Answer from the drawing. Dimensions are ordinates in mm from the lowest x, y and z of the part. Give positions to 0.01 mm unless a question says otherwise; leave off trailing zeros. Order: outer loops, then holes, each group sorted by start corner. A loop starts at its lowest first (then second) coordinate and runs counter-clockwise, first axis right, second up.
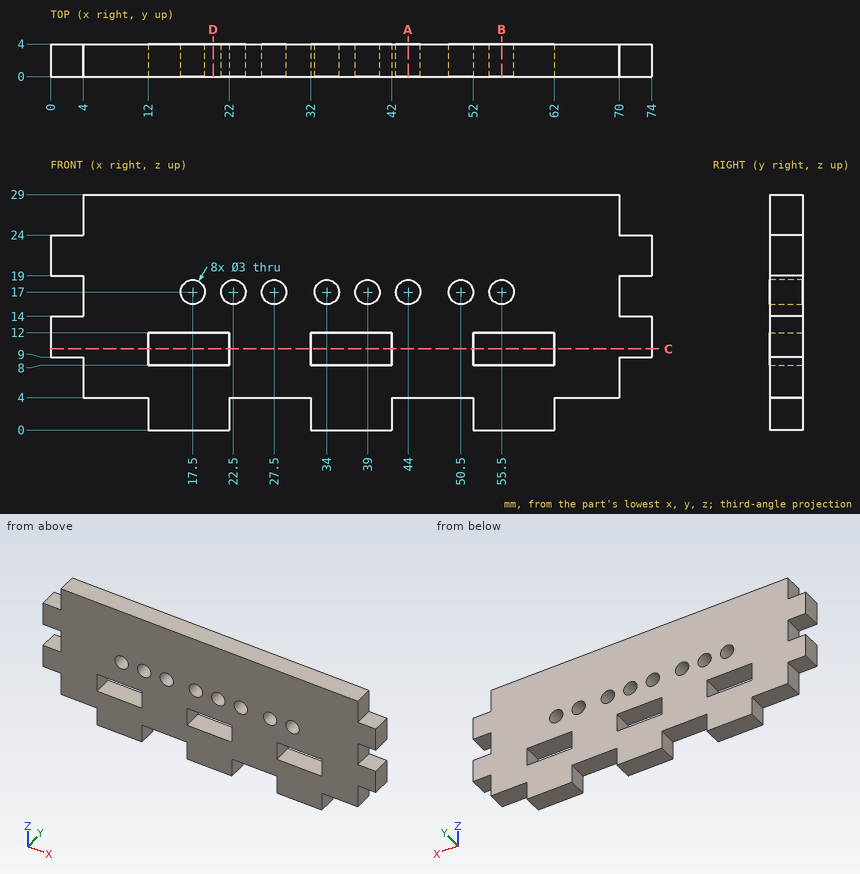
1. Straight lines are drawn through the part: probe 1 along X at (y, z) = (2, 10.75); probe 2 along Z at (x, y) = (61.5, 0.75); probe 3 along Z at (x, y) = (40, 2.75). For each, find the intervals that lie inside material, in ascending order.
Findings below:
probe 1: x = 0 to 12, 22 to 32, 42 to 52, 62 to 74
probe 2: z = 0 to 8, 12 to 29
probe 3: z = 0 to 8, 12 to 15.88, 18.12 to 29
2. The part is cut by section B-B (x = 55.5). Write down the section's boundary in (y, z), then the cut area to 3 significant figures.
Findings below:
outline: (0, 0) - (4, 0) - (4, 8) - (0, 8) - close; (0, 12) - (4, 12) - (4, 15.5) - (0, 15.5) - close; (0, 18.5) - (4, 18.5) - (4, 29) - (0, 29) - close
area: 88.0 mm2
3. The part is cut by section A-A (x = 44). Write down the section's boundary in (y, z).
Findings below:
outline: (0, 4) - (4, 4) - (4, 15.5) - (0, 15.5) - close; (0, 18.5) - (4, 18.5) - (4, 29) - (0, 29) - close
4. The part is cut by section C-C (z = 10). Write down the section's boundary in (x, y), then the cut area to 3 significant figures.
Findings below:
outline: (0, 0) - (12, 0) - (12, 4) - (0, 4) - close; (22, 0) - (32, 0) - (32, 4) - (22, 4) - close; (42, 0) - (52, 0) - (52, 4) - (42, 4) - close; (62, 0) - (74, 0) - (74, 4) - (62, 4) - close
area: 176 mm2
5. Given P1, Ø2.5, axis at x = 17.5, z = 17, coming from the -Y side; P2, Ø2, axis at x = 48, y = 1, coming from the -Z side; P3, Ø1.2, axis at y = 1, z = 6.5, coming from the -X side; P4, Ø2, axis at x = 72, y = 1.5, coming from the +Z side, each flat-ended and moving along its own axis, determine where each tip first touches the part or whether it passes through.
Findings below:
P1: passes through
P2: stops at z = 4
P3: stops at x = 4
P4: stops at z = 24
6. The part is cut by section D-D (x = 20). Write down the section's boundary in (y, z), then the cut area to 3 significant figures.
Findings below:
outline: (0, 0) - (4, 0) - (4, 8) - (0, 8) - close; (0, 12) - (4, 12) - (4, 29) - (0, 29) - close
area: 100 mm2
